from build123d import *

# Parameters (mm, degrees)
F0_W     = 52.410952
F0_H     = 44.566952
F0_R     = 11.883232
F1_DEPTH = 19.304
F2_R     = 4.74542
F3_DEPTH = 58.4708
F5_DEPTH = 25.4


with BuildPart() as f1:
    # F0 (on Top) → F1 (new body)
    with BuildSketch(Plane.XY):
        Rectangle(F0_W, F0_H)
        Circle(F0_R, mode=Mode.SUBTRACT)
    extrude(amount=F1_DEPTH)

    # F2 (on face) → F3 (cut)
    with BuildSketch(Plane.XZ.offset(22.283476)):
        with Locations((0, 10.076289)):
            Circle(F2_R)
    extrude(amount=-F3_DEPTH, mode=Mode.SUBTRACT)

    # F4 (on face) → F5 (cut)
    with BuildSketch(Plane.XY.offset(19.304)):
        Polygon((-15.993849, 12.278491), (-14.284679, 15.070137), (-14.769814, 18.307295), (-17.222254, 20.475263), (-20.494475, 20.559624), (-23.055369, 18.520906), (-23.706664, 15.313047), (-22.143613, 12.437039), (-19.097584, 11.2386), align=None)
    extrude(amount=-F5_DEPTH, mode=Mode.SUBTRACT)


solid = f1.part
For this review, take the finished solid that the model builds, in its own axes (mm). A direction names the side the tool comes from. Give positions to 0.01 mm unless a question says otherwise; leave off trailing zeros. Write each loop counter-clockwise with the first axis right and the second up, starting at its lowest first coordinate (ties: lowest second). Pieces come first, ordered by that corner, then holes. Notation, with made-up numbers: (-4, 86) -> (39, 86) arc R18 cw to (39, 93) -> close; hole circle Ø3 at (22.25, 83). An arc over 180 degrees is marked (long way). Use CSV: the item, a comma, the result in double quotes.
Q1. To check wall thickness, follow probe 1 along X at (y, z) = (17, 13); probe 2 along X at (y, z) = (-0.5, 14); probe 3 along Y at (x, z) = (-17, 6.25). State the ranges of each line that lie inside material, in increasing order. Write a range as [from, to].
Conclusion:
probe 1,"[-26.21, -23.36], [-14.57, -3.74], [3.74, 26.21]"
probe 2,"[-26.21, -11.87], [11.87, 26.21]"
probe 3,"[-22.28, 11.94], [20.28, 22.28]"
Q2. Take a section at C-C, the plane z = 12.75. Write out the cut boundary in (x, y).
Conclusion:
outline,"(-26.21, -22.28) -> (-3.92, -22.28) -> (-3.92, -11.22) arc R11.88 cw to (-3.92, 11.22) -> (-3.92, 22.28) -> (-26.21, 22.28) -> close; (3.92, -22.28) -> (26.21, -22.28) -> (26.21, 22.28) -> (3.92, 22.28) -> (3.92, 11.22) arc R11.88 cw to (3.92, -11.22) -> close; hole (-23.71, 15.31) -> (-22.14, 12.44) -> (-19.1, 11.24) -> (-15.99, 12.28) -> (-14.28, 15.07) -> (-14.77, 18.31) -> (-17.22, 20.48) -> (-20.49, 20.56) -> (-23.06, 18.52) -> close"
Q3. Mouldability with a two-part tool opening along X and no side actions: class faces 3 (the face through (-22.94, 13.9, 9.79)), 4 (the face through (26.205, 0, 10)), 5 (the face through (0, -22.283, 5)) as pulls with the +X half, pulls with the -X half, needs draft (parallel to the pull), parting line crosses it, or undercut.
Conclusion:
face 3,"undercut"
face 4,"pulls with the +X half"
face 5,"needs draft"
Q4. Take a section at D-D, the plane x = -10. Write out the cut boundary in (y, z).
Conclusion:
outline,"(-22.28, 0) -> (-6.42, 0) -> (-6.42, 19.3) -> (-22.28, 19.3) -> close; (6.42, 0) -> (22.28, 0) -> (22.28, 19.3) -> (6.42, 19.3) -> close"
Q5. Take a section at B-B, the plane y = 0. Write out the cut boundary in (x, z), then the cut area to 3 significant figures.
Conclusion:
outline,"(-26.21, 0) -> (-11.88, 0) -> (-11.88, 19.3) -> (-26.21, 19.3) -> close; (11.88, 0) -> (26.21, 0) -> (26.21, 19.3) -> (11.88, 19.3) -> close"
area,"553 mm2"
Q6. Tool access review of faces 1 (the face through (-20.642, 11.846, 9.787)), 2 (the face through (-4.74, 16.51, 10.28)): name each direction out of +Z, -Z, +X, -X, +Y, -Y from which nothing blocks a thin tool from reaching the whole face with its end or side.
Conclusion:
face 1,"+Z, -Z"
face 2,"+Y, -Y"
Q7. Take a section at A-A, the plane x = 0. Write out the cut boundary in (y, z), then the cut area to 3 significant figures.
Conclusion:
outline,"(-22.28, 0) -> (-11.88, 0) -> (-11.88, 5.33) -> (-22.28, 5.33) -> close; (-22.28, 14.82) -> (-11.88, 14.82) -> (-11.88, 19.3) -> (-22.28, 19.3) -> close; (11.88, 0) -> (22.28, 0) -> (22.28, 5.33) -> (11.88, 5.33) -> close; (11.88, 14.82) -> (22.28, 14.82) -> (22.28, 19.3) -> (11.88, 19.3) -> close"
area,"204 mm2"
